Could you check a few things on this drawing? It's one solid part, dimensions in mm from its lowest x, y, z. A direction names the side the tool comes from. Give positions to 0.01 mm unless a question says otherwise; leave off trailing zeros. Order: outer loops, then holes, each group sorted by start corner. A loop starts at its lowest first (then second) coordinate and runs counter-clockwise, first axis right, second up.
(1) Imagine slicing it at C-C, the plane z = 3.25. Write out the boundary of the cut face in (x, y) (3 decimals), then the cut area to 3 significant figures.
(2) Imagine slicing it at B-B, the plane y = 4.25. Write out the boundary of the cut face in (x, z), then the cut area to 3 significant figures.
(3) Imagine slicing it at A-A, the plane x = 3. Write out the boundary of the cut face in (y, z) (3 decimals).
(4) Will these pins go through, and if not, where does the flat tip stop? pin 1 (1.8 mm diameter, centred on x = 24, y = 6.5, fed in from -Z); pin 2 (3 mm diameter, centred on x = 3, y = 7.125, fed in from -Z); pin 3 (1.8 mm diameter, centred on y = 4.5, z = 0.5, fed in from +X).
(5) If I drill on probe 1 along Y at (x, z) = (3, 2.85) (3 decimals); probe 2 along X at (y, z) = (6, 2.2); probe 3 along Z at (x, y) = (3.75, 5.5), over which ranges is the centre line in solid material (lowest first)?
(6) On a 3-axis mill with a long thin cutter (end or side, diameter ignored), from which of +Z, -Z, +X, -X, +Y, -Y can I reach the whole of each face in a straight line? I mean the marked faces 1 and 2. Say none if no direction works.
(7) Imagine slicing it at D-D, the plane z = 0.5. Write out the boundary of the cut face in (x, y) (3 decimals).
(8) If we mould it in two halves opening along X, with no side actions, what happens to the marked faces 3 and 4? For each: released by +X, released by -X, zero draft, split by the parting line, or undercut.
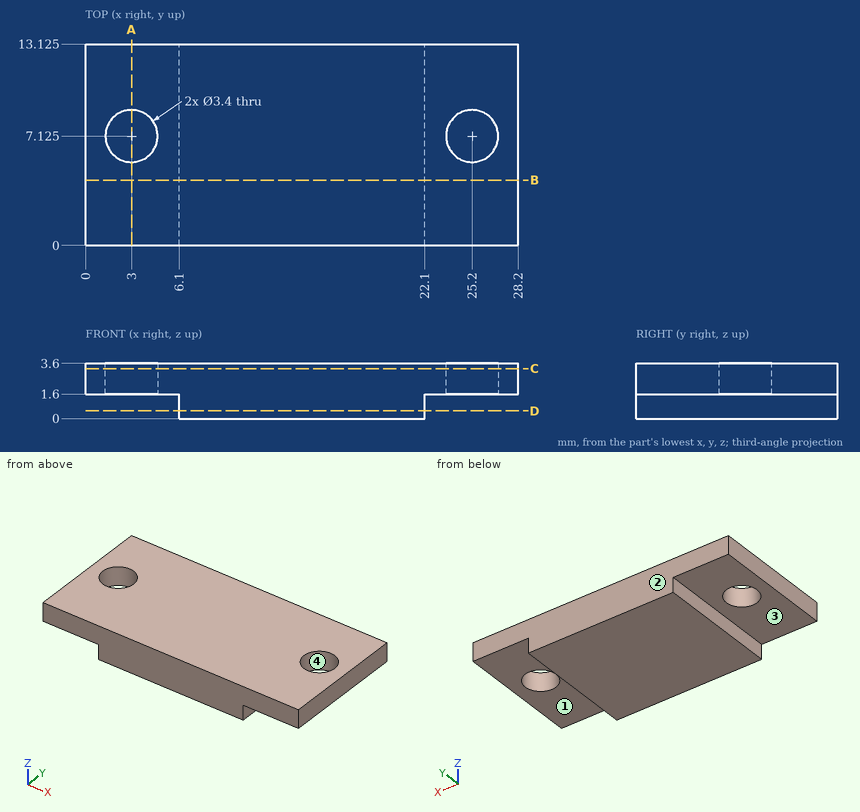
Answer block:
1. outline: (0, 0) - (28.2, 0) - (28.2, 13.125) - (0, 13.125) - close; hole circle Ø3.4 at (3, 7.125); hole circle Ø3.4 at (25.2, 7.125)
1. area: 352 mm2
2. outline: (0, 1.6) - (6.1, 1.6) - (6.1, 0) - (22.1, 0) - (22.1, 1.6) - (28.2, 1.6) - (28.2, 3.6) - (0, 3.6) - close
2. area: 82.0 mm2
3. outline: (0, 1.6) - (5.425, 1.6) - (5.425, 3.6) - (0, 3.6) - close; (8.825, 1.6) - (13.125, 1.6) - (13.125, 3.6) - (8.825, 3.6) - close
4. pin 1: stops at z = 1.6
4. pin 2: passes through
4. pin 3: stops at x = 22.1
5. probe 1: y = 0 to 5.425, 8.825 to 13.125
5. probe 2: x = 0 to 1.73, 4.27 to 23.93, 26.47 to 28.2
5. probe 3: z = 1.6 to 3.6
6. face 1: -Z, +X, +Y, -Y
6. face 2: +Z, -Z, +X, -X, +Y
7. outline: (6.1, 0) - (22.1, 0) - (22.1, 13.125) - (6.1, 13.125) - close
8. face 3: zero draft
8. face 4: undercut
